```python
from build123d import *

# Parameters (mm, degrees)
F0_R     = 6.35
F1_DEPTH = 25.4
F2_R     = 12.7
F3_R     = 12.7
F4_T     = -5.08
F6_R     = 10.7952537359
F5_DEPTH = 5.08


with BuildPart() as f1:
    # F0 (on Front) → F1 (new body)
    with BuildSketch(Plane.XZ):
        with BuildLine():
            Line((0, 63.5), (-36.1179809239, 63.5))
            ThreePointArc((-36.1179809239, 63.5), (-34.6565238325, 58.535797401), (-32.5163963302, 53.8242139571))
            ThreePointArc((-32.5163963302, 53.8242139571), (1.97e-08, 34.4563321571), (32.516396349, 53.8242139918))
            ThreePointArc((32.516396349, 53.8242139918), (34.6565238393, 58.5357974195), (36.1179809239, 63.5))
            Line((36.1179809239, 63.5), (0, 63.5))
        make_face()
        with BuildLine():
            Line((-36.1179809239, 63.5), (-50.8, 63.5))
            Line((-50.8, 63.5), (-50.8, -38.1))
            Line((-50.8, -38.1), (50.8, -38.1))
            Line((50.8, -38.1), (50.8, 63.5))
            Line((50.8, 63.5), (36.1179809239, 63.5))
            ThreePointArc((36.1179809239, 63.5), (34.6565238393, 58.5357974195), (32.516396349, 53.8242139918))
            ThreePointArc((32.516396349, 53.8242139918), (1.97e-08, 34.4563321571), (-32.5163963302, 53.8242139571))
            ThreePointArc((-32.5163963302, 53.8242139571), (-34.6565238325, 58.535797401), (-36.1179809239, 63.5))
        make_face()
        with Locations((-38.1, -25.4)):
            Circle(F0_R, mode=Mode.SUBTRACT)
        with Locations((38.1, -25.4)):
            Circle(F0_R, mode=Mode.SUBTRACT)
        with BuildLine():
            ThreePointArc((-31.75, 50.8), (-44.2554196974, 49.2400934809), (-32.5163963302, 53.8242139571))
            ThreePointArc((-32.5163963302, 53.8242139571), (-31.9445803026, 52.3599065191), (-31.75, 50.8))
        make_face(mode=Mode.SUBTRACT)
        with BuildLine():
            ThreePointArc((44.45, 50.8), (36.5400934618, 44.6445803074), (32.516396349, 53.8242139918))
            ThreePointArc((32.516396349, 53.8242139918), (39.6599065382, 56.9554196926), (44.45, 50.8))
        make_face(mode=Mode.SUBTRACT)
    extrude(amount=F1_DEPTH)

    # F2
    f2_edges = [f1.edges().sort_by_distance(p)[0] for p in [
        (-50.8, -12.7, -38.1),
        (50.8, -12.7, -38.1),
    ]]
    fillet(f2_edges, radius=F2_R)

    # F3
    f3_edges = [f1.edges().sort_by_distance(p)[0] for p in [
        (-50.8, -12.7, 63.5),
        (50.8, -12.7, 63.5),
    ]]
    fillet(f3_edges, radius=F3_R)

    # F4
    f4_openings = [f1.faces().sort_by_distance(p)[0] for p in [
        (0, -25.4, 12.7),
    ]]
    offset(amount=F4_T, openings=f4_openings, kind=Kind.INTERSECTION)

    # F6 (on face) → F5 (cut, through all)
    with BuildSketch(Plane.XZ):
        with Locations((0, 12.4445185065)):
            Circle(F6_R)
    extrude(amount=F5_DEPTH, mode=Mode.SUBTRACT)


solid = f1.part
```
Input: part model. Units: mm. Frame: model coordinates. A direction names the side the tool comes from. Coordinates: 2 decimals unless noted, no trailing zeros. Loops run counter-clockwise (first coordinate to the right, second up) from the corner with the lowest first, then second, coordinate; pieces in that order, holes last. Notation, with made-up numbers: (80, 64.5) -> (93, 64.5) arc R17 cw to (93, 87.5) -> close; hole circle Ø11 at (-11.5, 83.5). An arc over 180 degrees is marked (long way). Use a Markdown table: item, result.
1) Cut plane D-D (x = 0). Return the cut outline in (y, z), then the cut area to 3 significant figures.
Results found:
| item | result |
|---|---|
| outline | (-25.4, -38.1) -> (0, -38.1) -> (0, 1.65) -> (-5.08, 1.65) -> (-5.08, -33.02) -> (-25.4, -33.02) -> close; (-25.4, 58.42) -> (-5.08, 58.42) -> (-5.08, 23.24) -> (0, 23.24) -> (0, 63.5) -> (-25.4, 63.5) -> close |
| area | 613 mm2 |
2) Cut plane A-A (z = 8). Return the cut outline in (x, y), then the cut area to 3 significant figures.
Results found:
| item | result |
|---|---|
| outline | (-50.8, -25.4) -> (-45.72, -25.4) -> (-45.72, -5.08) -> (-9.84, -5.08) -> (-9.84, 0) -> (-50.8, 0) -> close; (9.84, -5.08) -> (45.72, -5.08) -> (45.72, -25.4) -> (50.8, -25.4) -> (50.8, 0) -> (9.84, 0) -> close |
| area | 623 mm2 |
3) Contact query for flat-ended pins moving along their axis: pin 1 (8 mm diameter, centred on x = 14, z = -25, fed in from -Y); pin 2 (4 mm diameter, centred on x = 24, z = -9, fed in from +Y); pin 3 (7.5 mm diameter, centred on x = 38.1, z = 50.8, fed in from +Y). Output: stop coordinate, or through.
Results found:
| item | result |
|---|---|
| pin 1 | stops at y = -5.08 |
| pin 2 | stops at y = 0 |
| pin 3 | passes through |
4) Access query for faces 1 (the cylindrical face through (46.98, -12.88, 59.88)), 2 (the flat face through (0, -15, 58.42)). Directions: +Z, -Z, +X, -X, +Y, -Y. A direction counts if a zero-diameter tool reaches every point of the face in a straight line with its end or side. Return the directions, or none.
Results found:
| item | result |
|---|---|
| face 1 | +Z, +X, +Y, -Y |
| face 2 | -Y |
5) Cut plane C-C (y = -23). Return the cut outline in (x, z), then the cut area to 3 significant figures.
Results found:
| item | result |
|---|---|
| outline | (-50.8, -25.4) arc R12.7 ccw to (-38.1, -38.1) -> (38.1, -38.1) arc R12.7 ccw to (50.8, -25.4) -> (50.8, 50.8) arc R12.7 ccw to (38.1, 63.5) -> (-38.1, 63.5) arc R12.7 ccw to (-50.8, 50.8) -> close; hole (-45.72, -16.88) arc R11.43 cw to (-29.58, -33.02) -> (29.58, -33.02) arc R11.43 cw to (45.72, -16.88) -> (45.72, 42.28) arc R11.43 cw to (29.58, 58.42) -> (-29.58, 58.42) arc R11.43 cw to (-45.72, 42.28) -> close; hole circle Ø12.7 at (-38.1, -25.4); hole circle Ø12.7 at (-38.1, 50.8); hole circle Ø12.7 at (38.1, -25.4); hole circle Ø12.7 at (38.1, 50.8) |
| area | 2,600 mm2 |
6) Material intervals for line 1 along Z through (x, y) = (-38.1, -11.75); line 2 along X through (y, z) = (-10.75, 46); line 3 along Z through (x, y) = (-4.5, -7.5), sorted ascending. Write a range as from..to.
Results found:
| item | result |
|---|---|
| line 1 | z = -38.1..-31.75, -19.05..-13.97, 39.37..44.45, 57.15..63.5 |
| line 2 | x = -50.8..-42.26, -33.94..-27.73, 27.73..33.94, 42.26..50.8 |
| line 3 | z = -38.1..-33.02, 58.42..63.5 |
7) Pull-direction query (X, two-part tool) for faces 3 (the cylindrical face through (-29.85, -15.1, -17.49)), 4 (the flat face through (-1, -13, -38.1)), 5 (the cylindrical face through (33.06, -12.52, -29.26)), 6 (the cylindrical face through (-47.18, -12.88, -34.28)); classes: released by +X, released by -X, zero draft, split by the parting line, or undercut.
Results found:
| item | result |
|---|---|
| face 3 | undercut |
| face 4 | zero draft |
| face 5 | undercut |
| face 6 | released by -X |
8) Cut plane B-B (x = 16.5). Return the cut outline in (y, z), then the cut area to 3 significant figures.
Results found:
| item | result |
|---|---|
| outline | (-25.4, -38.1) -> (0, -38.1) -> (0, 63.5) -> (-25.4, 63.5) -> (-25.4, 58.42) -> (-5.08, 58.42) -> (-5.08, -33.02) -> (-25.4, -33.02) -> close |
| area | 723 mm2 |
